For this review, take the finished solid that the model builds, in its own axes (mm). Face numbers are marked on the shaded views. A direction names the side the tool comes from. Coordinates: 2 decimals unless noted, no trailing zeros. Order: outer loops, then holes, each group sorted by start corner. A loop starts at its lowest first (then second) coordinate and runs counter-clockwise, first axis right, second up.
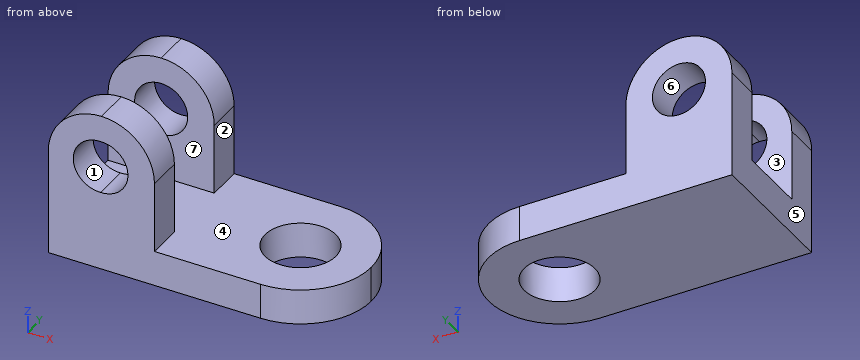
from build123d import *

# Parameters (mm, degrees)
F0_W      = 101.6
F0_H      = 50.8
F1_DEPTH  = 12.7
F3_R      = 25.39999
F2_R      = 12.7
F4_DEPTH  = 12.701
F5_W      = 38.1
F5_H      = 12.7
F6_DEPTH  = 44.45
F7_R      = 19.04999
F8_R      = 9.525
F9_DEPTH  = 50.801
F10_W     = 38.1
F10_H     = 12.7
F11_DEPTH = 44.45
F12_R     = 19.04999
F13_R     = 9.525
F14_DEPTH = 50.801


# Not quite as in the source:
# - a fillet or chamfer is up to 0.001 mm smaller than in the source, because OpenCascade refuses the exact size


with BuildPart() as f1:
    # F0 (on Top) → F1 (new body)
    with BuildSketch(Plane.XY):
        with Locations((11.9383526917, -1.5475824475)):
            Rectangle(F0_W, F0_H)
    extrude(amount=F1_DEPTH)

    # F3 (radius 25.4 in the source; OpenCascade refuses exactly that, so slightly less here)
    f3_edges = [f1.edges().sort_by_distance(p)[0] for p in [
        (62.738353, -26.947582, 6.35),
        (62.738353, 23.852418, 6.35),
    ]]
    fillet(f3_edges, radius=F3_R)

    # F2 (on face) → F4 (cut, through all)
    with BuildSketch(Plane.XY.offset(12.7)):
        with Locations((37.3383526917, -1.5475824475)):
            Circle(F2_R)
    extrude(amount=-F4_DEPTH, mode=Mode.SUBTRACT)

    # F5 (on face) → F6 (join)
    with BuildSketch(Plane.XY.offset(12.7)):
        with Locations((-19.8116473083, -20.5975824475)):
            Rectangle(F5_W, F5_H)
    extrude(amount=F6_DEPTH)

    # F7 (radius 19.05 in the source; OpenCascade refuses exactly that, so slightly less here)
    f7_edges = [f1.edges().sort_by_distance(p)[0] for p in [
        (-38.861647, -20.597582, 57.15),
        (-0.761647, -20.597582, 57.15),
    ]]
    fillet(f7_edges, radius=F7_R)

    # F8 (on face) → F9 (cut, through all)
    with BuildSketch(Plane.XZ.offset(26.9475824475)):
        with Locations((-20.3908979893, 38.1)):
            Circle(F8_R)
    extrude(amount=-F9_DEPTH, mode=Mode.SUBTRACT)

    # F10 (on face) → F11 (join)
    with BuildSketch(Plane.XY.offset(12.7)):
        with Locations((-19.8116473083, 17.5024175525)):
            Rectangle(F10_W, F10_H)
    extrude(amount=F11_DEPTH)

    # F12 (radius 19.05 in the source; OpenCascade refuses exactly that, so slightly less here)
    f12_edges = [f1.edges().sort_by_distance(p)[0] for p in [
        (-0.761647, 17.502418, 57.15),
        (-38.861647, 17.502418, 57.15),
    ]]
    fillet(f12_edges, radius=F12_R)

    # F13 (on face) → F14 (cut, through all)
    with BuildSketch(Plane(origin=(0, 23.8524175525, 0), x_dir=(-1, 0, 0), z_dir=(0, 1, 0))):
        with Locations((19.8116473083, 38.1)):
            Circle(F13_R)
    extrude(amount=-F14_DEPTH, mode=Mode.SUBTRACT)


solid = f1.part
1. Clearance check with flat-ended pins moving along their axes: pin 1 Ø8 at (y, z) = (7.5, 26.5) entering from +X; pin 2 Ø2 at (x, y) = (-6, -6.5) entering from +Z; pin 3 Ø10 at (x, y) = (-7.5, 15.5) entering from +Z. State where each tip first meets the part, or that it passes through.
Answer below:
pin 1: stops at x = -0.76
pin 2: stops at z = 12.7
pin 3: stops at z = 55.69
2. Take a section at C-C, the plane z = 40.5. Give the boundary of the cut face in (x, y), plus the area to 3 significant figures.
Answer below:
outline: (-38.71, -26.95) - (-29.61, -26.95) - (-29.61, -14.25) - (-38.71, -14.25) - close; (-38.71, 11.15) - (-29.03, 11.15) - (-29.03, 23.85) - (-38.71, 23.85) - close; (-10.59, -26.95) - (-0.91, -26.95) - (-0.91, -14.25) - (-10.59, -14.25) - close; (-10.59, 11.15) - (-0.91, 11.15) - (-0.91, 23.85) - (-10.59, 23.85) - close
area: 484 mm2
3. Machinability: for the marked faces 1, 2, 3 and 4, which of the approach directions +Z, -Z, +X, -X, +Y, -Y give a long, thin tool a straight path to every point of the face, cutting with its end or side? Answer none if there is none.
Answer below:
face 1: -Y
face 2: +Z, +X, +Y, -Y
face 3: +Z, +X, -X
face 4: +Z, +X
4. Take a section at D-D, the plane x = -15.5. Give the boundary of the cut face in (y, z).
Answer below:
outline: (-26.95, 0) - (23.85, 0) - (23.85, 29.61) - (11.15, 29.61) - (11.15, 12.7) - (-14.25, 12.7) - (-14.25, 29.61) - (-26.95, 29.61) - close; (-26.95, 46.59) - (-14.25, 46.59) - (-14.25, 56.66) - (-26.95, 56.66) - close; (11.15, 46.59) - (23.85, 46.59) - (23.85, 56.66) - (11.15, 56.66) - close
5. The part is to be moulded in two halves that separate along X. For the marked faces 5, 6 and 7, say which applies: +X half, -X half, draft (parallel to the pull), parting line (faces both ways), or undercut.
Answer below:
face 5: -X half
face 6: undercut
face 7: draft
6. To check wall thickness, follow L1, parallel to X at y = 15, z = 38; L2, parallel to Y at x = -22, z = 22; L3, parallel to Z at x = 4.5, y = -23.5. State the ranges of each line that lie inside material, in increasing order.
Answer below:
L1: x = -38.86 to -29.34, -10.29 to -0.76
L2: y = -26.95 to -14.25, 11.15 to 23.85
L3: z = 0 to 12.7
7. Take a section at A-A, the plane z = 52. Give the boundary of the cut face in (x, y).
Answer below:
outline: (-32.84, -26.95) - (-6.79, -26.95) - (-6.79, -14.25) - (-32.84, -14.25) - close; (-32.84, 11.15) - (-6.79, 11.15) - (-6.79, 23.85) - (-32.84, 23.85) - close
